Geometry: final body of the model. Coordinates: model frame, mm. A direction names the side the tool comes from. Give positions to 0.01 mm unless a question says otherwise; leave off trailing zeros. Order: outer loops, then holes, each group sorted by start corner. A loop starts at its lowest first (then second) coordinate and runs counter-clockwise, first axis right, second up. Notation, with made-up numbers: (28, -1.75) - (50, -1.75) arc R7 cw to (50, 10.25) - close; hole circle Ø10 at (65.5, 16). An arc over 180 degrees is marked (long way). Put each result on its own line as item: value. Start each with the question number.
1. Section D-D on y = -15.5. Return the cut outline in (x, z) (3 decimals), plus the area to 3 significant figures.
2. Ray query, line 1 along Z through (x, y) = (11.5, 55) (3 decimals); line 2 along Y through (x, z) = (27, 24); line 3 along Y through (x, z) = (16.5, 30.5). Return the intervals inside material, ascending. Write a range as from..to.
3. Mould query, pull axis Z, two halves, no side actions, for faces 1 (the flat face through (0, -7.938, 35)), 2 (the flat face through (1, 35, 9.525)), 3 (the flat face through (-1, -1, -9.525)). Classes: pulls with the +Z half, pulls with the -Z half, needs draft (parallel to the pull), parting line crosses it, or undercut.
4. Set-up query: faces 4 (the flat face through (94, 0, 48.129)), 5 (the flat face through (1, -36, 9.525)), 6 (the flat face through (50, -25.4, 55)). Return all of +Z, -Z, +X, -X, +Y, -Y with unobstructed straight access to the full face (end or side cutting, diameter ignored); none if empty.
5. First-contact query: P1, Ø8, axis at x = 43.5, y = 47.5, coming from the +Z side (3 decimals); P2, Ø12, axis at x = 78.5, z = 60, coming from the +Y side; P3, Ø1.5, axis at x = -5, z = 32, coming from the +Y side. Flat tips, straight axial feed; report the tip coordinate or a pass-through.
6. Section A-A on z = -2.5. Return the cut outline in (x, y) (3 decimals), plus the area to 3 significant figures.
7. Section C-C on y = -33.5. Return the cut outline in (x, z) (3 decimals), plus the area to 3 significant figures.
8. Section B-B on y = 22.5. Return the cut outline in (x, z) (3 decimals), plus the area to 3 significant figures.
from build123d import *

# Parameters (mm, degrees)
F1_DEPTH = 63.5
F0_W     = 26.0042664987
F0_H     = 17.5260005385
F2_DEPTH = 25.4
F3_DEPTH = 7.9375
F5_R     = 5.08


with BuildPart() as f1:
    # F0 (on Front) → F1 (new body, symmetric)
    with BuildSketch(Plane.XZ):
        Polygon((23.7489994615, 9.525), (-41.275, 9.525), (-41.275, -9.525), (41.275, -9.525), (41.275, 9.525), align=None)
    extrude(amount=F1_DEPTH, both=True)

    # F0 (on Front) → F2 (join, symmetric)
    with BuildSketch(Plane.XZ):
        with BuildLine():
            Line((23.7489994615, 38.1957218051), (23.7489994615, 9.525))
            Line((23.7489994615, 9.525), (41.275, 9.525))
            Line((41.275, 9.525), (41.275, 38.1957218051))
            ThreePointArc((41.275, 38.1957218051), (46.1106670426, 49.8700547625), (57.785, 54.7057218051))
            Line((57.785, 54.7057218051), (67.6709335013, 54.7057218051))
            Line((67.6709335013, 54.7057218051), (67.6709335013, 72.2317223436))
            Line((67.6709335013, 72.2317223436), (62.7786442637, 72.2317223436))
            Line((62.7786442637, 72.2317223436), (57.785, 72.2317223436))
            ThreePointArc((57.785, 72.2317223436), (33.7179132148, 62.2628085903), (23.7489994615, 38.1957218051))
        make_face()
        with Locations((80.6730667507, 63.4687220743)):
            Rectangle(F0_W, F0_H)
    extrude(amount=F2_DEPTH, both=True)

    # F0 (on Front) → F3 (join, symmetric)
    with BuildSketch(Plane.XZ):
        with BuildLine():
            add(Edge.make_bspline(
                [(-41.275, 9.525), (-35.4608595371, 69.9300542474), (14.8590393364, 73.8207250834), (62.7786442637, 72.2317223436)],
                knots=[0, 0, 0, 0, 121.4878344183, 121.4878344183, 121.4878344183, 121.4878344183], degree=3))
            Line((-41.275, 9.525), (23.7489994615, 9.525))
            Line((23.7489994615, 9.525), (23.7489994615, 38.1957218051))
            ThreePointArc((23.7489994615, 38.1957218051), (33.7179132148, 62.2628085903), (57.785, 72.2317223436))
            Line((57.785, 72.2317223436), (62.7786442637, 72.2317223436))
        make_face()
    extrude(amount=F3_DEPTH, both=True)

    # F0 (on Front) → F4 (revolve)
    with BuildSketch(Plane.XZ):
        Polygon((93.6752, 76.7040487946), (93.6752, 72.2317223436), (93.6752, 54.7057218051), (93.6752, 48.1290487946), (118.4709335013, 48.1290487946), (118.4709335013, 76.7040487946), align=None)
    revolve(axis=Axis((93.6752, 0, 62.4165487946), (0, 0, 1)))

    # F5
    f5_edges = [f1.edges().sort_by_distance(p)[0] for p in [
        (41.275, 63.5, 0),
        (-41.275, 63.5, 0),
        (-41.275, -63.5, 0),
        (41.275, -63.5, 0),
    ]]
    fillet(f5_edges, radius=F5_R)


solid = f1.part
Resolved:
1. outline: (-41.275, -9.525) - (41.275, -9.525) - (41.275, 38.196) arc R16.51 cw to (57.785, 54.706) - (74.321, 54.706) - (74.321, 48.129) - (113.029, 48.129) - (113.029, 76.704) - (74.321, 76.704) - (74.321, 72.232) - (57.785, 72.232) arc R34.036 ccw to (23.749, 38.196) - (23.749, 9.525) - (-41.275, 9.525) - close
1. area: 4,170 mm^2
2. line 1: -9.525..9.525
2. line 2: -25.4..25.4
2. line 3: -7.94..7.94
3. face 1: needs draft
3. face 2: pulls with the +Z half
3. face 3: pulls with the -Z half
4. face 4: -Z, +X, +Y, -Y
4. face 5: +Z, -X, -Y
4. face 6: +Z, +X, -X, -Y
5. P1: z = 9.525
5. P2: y = 25.4
5. P3: y = 7.94
6. outline: (-41.275, -58.42) arc R5.08 ccw to (-36.195, -63.5) - (36.195, -63.5) arc R5.08 ccw to (41.275, -58.42) - (41.275, 58.42) arc R5.08 ccw to (36.195, 63.5) - (-36.195, 63.5) arc R5.08 ccw to (-41.275, 58.42) - close
6. area: 10,500 mm^2
7. outline: (-41.275, -9.525) - (41.275, -9.525) - (41.275, 9.525) - (-41.275, 9.525) - close
7. area: 1,570 mm^2
8. outline: (-41.275, -9.525) - (41.275, -9.525) - (41.275, 38.196) arc R16.51 cw to (57.785, 54.706) - (83.255, 54.706) - (83.255, 48.129) - (104.095, 48.129) - (104.095, 76.704) - (83.255, 76.704) - (83.255, 72.232) - (57.785, 72.232) arc R34.036 ccw to (23.749, 38.196) - (23.749, 9.525) - (-41.275, 9.525) - close
8. area: 3,810 mm^2
